The drawing under review shows one solid part. Ordinate dimensions are in mm from its lowest x, y, z. A direction names the side the tool comes from. Give positions to 0.01 mm unless a question says otherwise; leave off trailing zeros. Order: outer loops, then holes, each group sorted by start corner. A loop starts at its lowest first (then second) coordinate and runs counter-clockwise, first axis right, second up. Notation, with made-up numbers: (13.5, 2) -> (41.5, 2) arc R20 ccw to (41.5, 25) -> close; hole circle Ø8 at (-9, 22). An arc over 180 degrees is marked (long way). Return JSON: item names as keys, results as strings. Group by question number.
1) Add section A-A (x = 22). Give the boundary of the cut face in (y, z).
2) Add section C-C (z = 5). Give the boundary of the cut face in (x, y).
3) Add section B-B (y = 3.75). Give the boundary of the cut face in (x, z), then the cut area to 3 significant figures.
4) Insertion check: P1, Ø0.7, axis at x = 22.5, y = 3.5, coming from the +Z side; P2, Ø5, axis at x = 6.5, z = 20.5, coming from the -Y side; P3, Ø1.5, axis at y = 2.5, z = 15.5, coming from the -X side; P4, Ø1, axis at x = 23.5, z = 15, coming from the -Y side. Each pin has a flat end and moves straight along its axis. Give the tip position at first contact, or say it passes through.
5) For the marked faces 1 and 2, list the 3-axis set-ups (+Z, -Z, +X, -X, +Y, -Y) from which the entire face can be reached by the end or side of a thin tool; tool diameter is ignored.
6) Add section D-D (x = 5.25). Give the boundary of the cut face in (y, z), then the cut area to 3 significant figures.
7) To check wall thickness, follow line 1 along Y through (x, z) = (22, 24.25); line 2 along X through (y, z) = (3, 4); line 3 along Z through (x, y) = (10, 0.75). State the ranges of each line that lie inside material, in increasing order.
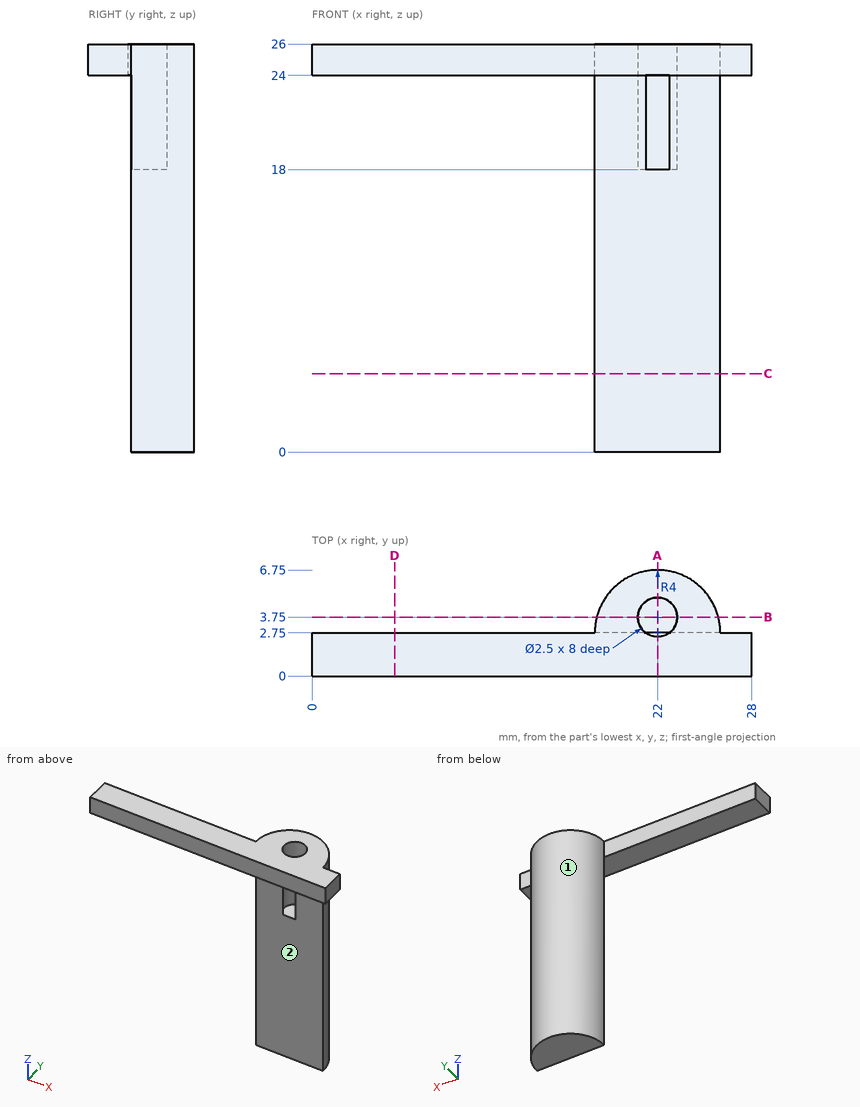
Evaluation:
{
 "1": {"outline": "(0, 24) -> (2.5, 24) -> (2.5, 26) -> (0, 26) -> close; (2.75, 0) -> (6.75, 0) -> (6.75, 26) -> (5, 26) -> (5, 18) -> (2.75, 18) -> close"},
 "2": {"outline": "(18, 2.75) -> (26, 2.75) arc R4 ccw to start"},
 "3": {"outline": "(18.13, 0) -> (25.87, 0) -> (25.87, 26) -> (23.25, 26) -> (23.25, 18) -> (20.75, 18) -> (20.75, 26) -> (18.13, 26) -> close", "area": "181 mm^2"},
 "4": {"P1": "z = 18", "P2": "through", "P3": "x = 18", "P4": "y = 2.75"},
 "5": {"face 1": "+Z, -Z, +Y", "face 2": "-Z, +X, -X, -Y"},
 "6": {"outline": "(0, 24) -> (2.75, 24) -> (2.75, 26) -> (0, 26) -> close", "area": "5.50 mm^2"},
 "7": {"line 1": "0 to 2.5, 5 to 6.75", "line 2": "18.01 to 25.99", "line 3": "24 to 26"}
}
